Verification items for the finished model (mm, model axes). A direction names the side the tool comes from. Give positions to 0.01 mm unless a question says otherwise; leave off trailing zeros. Write each loop counter-clockwise with the first axis right and the second up, starting at its lowest first coordinate (ties: lowest second). Pieces come first, ordered by that corner, then holes. Notation, with made-up numbers: M 81,-11.5 L 126,-11.5 A16 ccw 126,12.5 Z; hole C -40,22.5 d3. An arc over 180 degrees is marked long. Answer as a JSON object with one key per item and string values.
```python
from build123d import *

# Parameters (mm, degrees)
SKETCH1_R      = 13.875
EXTRUDE1_DEPTH = 20.85
SKETCH3_R      = 4.45
EXTRUDE2_DEPTH = 2
EXTRUDE3_DEPTH = 2.75
SKETCH6_R      = 1.575
EXTRUDE4_DEPTH = 8.4
EXTRUDE5_START = 1.4
SKETCH7_R      = 1.575
EXTRUDE5_DEPTH = 1.4
SKETCH8_R      = 1.2
EXTRUDE7_DEPTH = 3


with BuildPart() as part:
    # Sketch1 → Extrude1 (new body)
    with BuildSketch(Plane(origin=(0, 0, 0), x_dir=(1, 0, 0), z_dir=(0, 1, 0))):
        with Locations(Location((0, 0, 0), (0, 0, 270))):
            Circle(SKETCH1_R)
    extrude(amount=EXTRUDE1_DEPTH)

    # Sketch2 → Cut-Revolve1 (revolve, cut)
    with BuildSketch(Plane.XY, mode=Mode.PRIVATE) as cut_revolve1_sk:
        Polygon((8.35, 20.85), (13.875, 17.4), (13.875, 20.85), align=None)
    revolve(cut_revolve1_sk.sketch.rotate(Axis((0, 20.85, 0), (0, -1, 0)), 90), axis=Axis((0, 20.85, 0), (0, -1, 0)), mode=Mode.SUBTRACT)

    # Sketch3 → Extrude2 (add)
    with BuildSketch(Plane(origin=(0, 20.85, 0), x_dir=(1, 0, 0), z_dir=(0, 1, 0))):
        with Locations(Location((0, 0, 0), (0, 0, 270))):
            Circle(SKETCH3_R)
    extrude(amount=EXTRUDE2_DEPTH)

    # Sketch4 → Extrude3 (cut)
    with BuildSketch(Plane.XZ):
        with BuildLine():
            ThreePointArc((-13.518505835, 3.125), (-6.169187379, 6.169187379), (-3.125, 13.518505835))
            ThreePointArc((-3.125, 13.518505835), (-9.811106589, 9.811106589), (-13.518505835, 3.125))
        make_face()
        with BuildLine():
            ThreePointArc((3.125, 13.518505835), (6.169187379, 6.169187379), (13.518505835, 3.125))
            ThreePointArc((13.518505835, 3.125), (9.811106589, 9.811106589), (3.125, 13.518505835))
        make_face()
        with BuildLine():
            ThreePointArc((13.518505835, -3.125), (6.169187379, -6.169187379), (3.125, -13.518505835))
            ThreePointArc((3.125, -13.518505835), (9.811106589, -9.811106589), (13.518505835, -3.125))
        make_face()
        with BuildLine():
            ThreePointArc((-3.125, -13.518505835), (-6.169187379, -6.169187379), (-13.518505835, -3.125))
            ThreePointArc((-13.518505835, -3.125), (-9.811106589, -9.811106589), (-3.125, -13.518505835))
        make_face()
    extrude(amount=-EXTRUDE3_DEPTH, mode=Mode.SUBTRACT)

    # Sketch5 → Cut-Revolve2 (revolve, cut)
    with BuildSketch(Plane(origin=(0, 0, 0), x_dir=(0, 0, -1), z_dir=(1, 0, 0))):
        Polygon((-13.875, 0), (-12.375, 0), (-13.875, 6), align=None)
    revolve(axis=Axis((0, 20.85, 0), (0, -1, 0)), mode=Mode.SUBTRACT)

    # Sketch6 → Extrude4 (add)
    with BuildSketch(Plane(origin=(0, 22.85, 0), x_dir=(-1, 0, 0), z_dir=(0, 1, 0))):
        with Locations(Location((0, 0, 0), (0, 0, 90))):
            Circle(SKETCH6_R)
    extrude(amount=EXTRUDE4_DEPTH)

    # Sketch7 → Extrude5 (add)
    with BuildSketch(Plane.XZ.offset(EXTRUDE5_START)):
        with Locations(Location((0, 0, 0), (0, 0, 90))):
            Circle(SKETCH7_R)
    extrude(amount=-EXTRUDE5_DEPTH)

    # Sketch8 → Extrude7 (cut)
    with BuildSketch(Plane.XZ):
        with Locations(Location((-7.95, 0, 0), (0, 0, 270))):
            Circle(SKETCH8_R)
        with Locations(Location((7.95, 0, 0), (0, 0, 270))):
            Circle(SKETCH8_R)
        with Locations(Location((0, 9.45, 0), (0, 0, 270))):
            Circle(SKETCH8_R)
        with Locations(Location((0, -9.45, 0), (0, 0, 270))):
            Circle(SKETCH8_R)
    extrude(amount=-EXTRUDE7_DEPTH, mode=Mode.SUBTRACT)


solid = part.part
```
1) Thickness scan on L1, parallel to X at y = 2.3, z = 0; L2, parallel to X at y = 1.8, z = -9.45; L3, parallel to Y at x = 2, z = -6. Record the ranges inside material, lowest first.
Completed:
{"L1": "x = -12.95 to -9.15, -6.75 to 6.75, 9.15 to 12.95", "L2": "x = -3.95 to -1.2, 1.2 to 3.95", "L3": "y = 0 to 20.85"}
2) Release check for a two-part mould opening along X. For faces 1 (the face through (6.1, 1.36, 6.24)), 2 (the face through (0, -1.4, 0)), 3 (the face through (-6.76, 1.48, 0.16)) record: pulls with the +X half, pulls with the -X half, needs draft (parallel to the pull), parting line crosses it, or undercut.
Completed:
{"face 1": "pulls with the +X half", "face 2": "needs draft", "face 3": "undercut"}
3) Go/stop test with flat-tipped pins: pin 1 (1 mm diameter, centred on x = 3.5, y = 21, fed in from -Z); pin 2 (12 mm diameter, centred on y = 10, z = -9.5, fed in from -X); pin 3 (6 mm diameter, centred on x = -6.5, z = 9.5, fed in from +Y); pin 4 (5 mm diameter, centred on x = -5, y = 28, fed in from -Z). Record where each tip stops, or that it passes through.
Completed:
{"pin 1": "stops at z = -8.22", "pin 2": "stops at x = -13.43", "pin 3": "stops at y = 20.75", "pin 4": "passes through"}
4) Section check D-D on y = 20. Record the boundary of the cut face in (x, z), and give its area (3 significant figures).
Completed:
{"outline": "C 0,0 d19.42", "area": "296 mm2"}
5) Section check A-A on z = 0. Record the boundary of the cut face in (x, y) (3 decimals), and give its area (3 significant figures).
Completed:
{"outline": "M -13.875,6 L -12.375,0 L -9.15,0 L -9.15,3 L -6.75,3 L -6.75,0 L -1.575,0 L -1.575,-1.4 L 1.575,-1.4 L 1.575,0 L 6.75,0 L 6.75,3 L 9.15,3 L 9.15,0 L 12.375,0 L 13.875,6 L 13.875,17.4 L 8.35,20.85 L 4.45,20.85 L 4.45,22.85 L 1.575,22.85 L 1.575,31.25 L -1.575,31.25 L -1.575,22.85 L -4.45,22.85 L -4.45,20.85 L -8.35,20.85 L -13.875,17.4 Z", "area": "585 mm2"}
6) Access from +Z, -Z, +X, -X, +Y, -Y to the whole of each face (thin tool, end or side, straight path). Record for faces 4 (the face through (-6.24, 1.36, 6.1)), 5 (the face through (3.01, 21.84, -3.28)), 6 (the face through (0.36, 1.479, 8.305)), 7 (the face through (8, 2.75, 8)), 8 (the face through (6.24, 1.36, -6.1)).
Completed:
{"face 4": "+Z, -X, -Y", "face 5": "+Y", "face 6": "-Y", "face 7": "+Z, +X, -Y", "face 8": "-Z, +X, -Y"}
7) Section check B-B on x = 0. Record the boundary of the cut face in (y, z) (3 decimals), and give its area (3 significant figures).
Completed:
{"outline": "M -1.4,-1.575 L 0,-1.575 L 0,-8.25 L 3,-8.25 L 3,-10.65 L 0,-10.65 L 0,-12.375 L 6,-13.875 L 17.4,-13.875 L 20.85,-8.35 L 20.85,-4.45 L 22.85,-4.45 L 22.85,-1.575 L 31.25,-1.575 L 31.25,1.575 L 22.85,1.575 L 22.85,4.45 L 20.85,4.45 L 20.85,8.35 L 17.4,13.875 L 6,13.875 L 0,12.375 L 0,10.65 L 3,10.65 L 3,8.25 L 0,8.25 L 0,1.575 L -1.4,1.575 Z", "area": "585 mm2"}
8) Section check C-C on y = 27. Record the boundary of the cut face in (x, z) (3 decimals).
Completed:
{"outline": "C 0,0 d3.15"}
